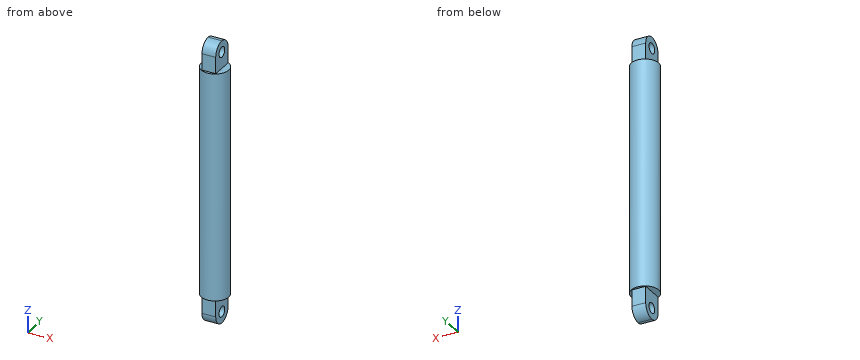
Autodesk Inventor part; units mm, degrees
ref_plane "YZ Plane" through (0, 0, 0) normal (1, 0, 0) x (0, 1, 0)
ref_plane "XZ Plane" through (0, 0, 0) normal (0, 1, 0) x (-1, 0, 0)
ref_plane "XY Plane" through (0, 0, 0) normal (0, 0, 1) x (1, 0, 0)
sketch "Sketch1" plane through (0, 0, 0) normal (0, 0, 1) x (1, 0, 0)
  circle A0 centre (0, 0) radius 25.4
  dimension "d0" = 50.8
extrude "Extrusion1" add sketch "Sketch1" along normal mid plane 419.1
sketch "Sketch4" plane through (0, 0, 209.55) normal (0, 0, 1) x (1, 0, 0)
  line L0 (-12.7, 20.6375) -> (12.7, 20.6375)
  line L1 (12.7, 20.6375) -> (12.7, -20.6375)
  line L2 (12.7, -20.6375) -> (-12.7, -20.6375)
  line L3 (-12.7, -20.6375) -> (-12.7, 20.6375)
  line L4 (-12.7, 20.6375) -> (12.7, -20.6375) construction
  line L5 (12.7, 20.6375) -> (-12.7, -20.6375) construction
  point P0 (0, 0)
  dimension "d15" = 25.4
  dimension "d16" = 41.275
extrude "Extrusion4" add sketch "Sketch4" along normal blind 50.8
fillet "Fillet2" radius 20.6375 2 edges at (0, 20.6375, 260.35) (0, -20.6375, 260.35)
sketch "Sketch5" plane through (12.7, -20.6375, 209.55) normal (1, 0, 0) x (0, 0, -1)
  arc A0 (-30.1625, 41.275) -> (-30.1625, 0) centre (-30.1625, 20.6375) ccw
  circle A1 centre (-30.1625, 20.6375) radius 9.525
  point P0 (209.55, 20.6375)
extrude "Extrusion5" cut sketch "Sketch5" against normal blind 50.8
mirror "Mirror1" about plane through (0, 0, 0) normal (0, 0, 1) of "Extrusion4", "Fillet2", "Extrusion5"
properties part number "body to wheel hub connectors (22 in)"
Design review of the part built by this model. Coordinates are the model's own, in mm. Coordinates: 2 decimals unless noted, no trailing zeros. Loops run counter-clockwise (first coordinate to the right, second up) from the corner with the lowest first, then second, coordinate; pieces in that order, holes last.
Item 1: Add section D-D (z = -218.5). Write out the cut boundary in (x, y).
Completed:
outline: (-12.7, -20.64) - (12.7, -20.64) - (12.7, 20.64) - (-12.7, 20.64) - close
Item 2: Add section B-B (y = -15.5). Write out the cut boundary in (x, z), and give its area (3 significant figures).
Completed:
outline: (-20.12, -209.55) - (-12.7, -209.55) - (-12.7, -253.34) - (12.7, -253.34) - (12.7, -209.55) - (20.12, -209.55) - (20.12, 209.55) - (12.7, 209.55) - (12.7, 253.34) - (-12.7, 253.34) - (-12.7, 209.55) - (-20.12, 209.55) - close
area: 19,100 mm2
Item 3: Add section A-A (x = 0). Give the number of separate pieces and of enclosed holes in the cut face, and give its area (3 significant figures).
Completed:
separate pieces: 1
enclosed holes: 2
area: 24,500 mm2
Item 4: Add section C-C (z = -27). Write out the cut boundary in (x, y), and give its area (3 significant figures).
Completed:
outline: circle Ø50.8 at (0, 0)
area: 2,030 mm2
Item 5: Clearance check with flat-ended pins moving along their axes: pin 1 (7.5 mm diameter, centred on x = 2.5, z = 218.5, fed in from +Y); pin 2 (10 mm diameter, centred on y = 11, z = -170.5, fed in from +X); pin 3 (20.5 mm diameter, centred on y = 10, z = -223.5, fed in from +X); pin 4 (15 mm diameter, centred on y = 0, z = -239.71, fed in from -X). State where each tip first meets the part, or that it passes through.
Completed:
pin 1: stops at y = 20.64
pin 2: stops at x = 24.68
pin 3: stops at x = 12.7
pin 4: passes through
Item 6: Wall thickness on L1, parallel to Z at x = 10, y = 1; L2, parallel to Z at x = 7, y = -6.5; L3, parallel to Y at x = 0, z = -197: over which ranges is each line inside the solid? List them lowest first.
Completed:
L1: z = -260.33 to -249.18, -230.24 to 230.24, 249.18 to 260.33
L2: z = -259.3 to -246.67, -232.75 to 232.75, 246.67 to 259.3
L3: y = -25.4 to 25.4
